Design review of the part built by this model. Coordinates are the model's own, in mm. Coordinates: 2 decimals unless noted, no trailing zeros. Loops run counter-clockwise (first coordinate to the right, second up) from the corner with the lowest first, then second, coordinate; pieces in that order, holes last. Notation, with made-up numbers: M 41.5,69 L 47.5,69 A12 cw 47.5,82 Z; hole C 13,50.5 d6. An arc over 180 degrees is marked long. Write item = value, one per line. Start each with the question number.
from build123d import *

# Parameters (mm, degrees)
SKETCH1_R               = 75.8825
BOSS_EXTRUDE1_DEPTH     = 38.1
SKETCH2_R               = 73.66
CUT_EXTRUDE1_DEPTH      = 101.6
SKETCH4_R               = 1.27
CUT_EXTRUDE3_DEPTH      = 76.8825
CUT_EXTRUDE3_DEPTH_BACK = 76.8825
SKETCH5_R               = 1.27
CUT_EXTRUDE4_DEPTH      = 76.8825001
CUT_EXTRUDE4_DEPTH_BACK = 76.8825001


with BuildPart() as part:
    # Sketch1 → Boss-Extrude1 (new body)
    with BuildSketch(Plane(origin=(0, 0, 0), x_dir=(1, 0, 0), z_dir=(0, 1, 0))):
        Circle(SKETCH1_R)
    extrude(amount=BOSS_EXTRUDE1_DEPTH)

    # Sketch2 → Cut-Extrude1 (cut)
    with BuildSketch(Plane(origin=(0, 38.1, 0), x_dir=(1, 0, 0), z_dir=(0, 1, 0))):
        Circle(SKETCH2_R)
    extrude(amount=-CUT_EXTRUDE1_DEPTH, mode=Mode.SUBTRACT)

    # Sketch4 → Cut-Extrude3 (cut, two sides)
    with BuildSketch(Plane(origin=(0, 0, 0), x_dir=(0, 0, -1), z_dir=(1, 0, 0))) as cut_extrude3_sk:
        with Locations((4.12e-07, 22.606)):
            Circle(SKETCH4_R)
        with Locations((4.12e-07, 15.494)):
            Circle(SKETCH4_R)
    extrude(amount=CUT_EXTRUDE3_DEPTH, mode=Mode.SUBTRACT)
    extrude(cut_extrude3_sk.sketch, amount=-CUT_EXTRUDE3_DEPTH_BACK, mode=Mode.SUBTRACT)

    # Sketch5 → Cut-Extrude4 (cut, two sides)
    with BuildSketch(Plane.XY) as cut_extrude4_sk:
        with Locations((7.8e-08, 15.493965738)):
            Circle(SKETCH5_R)
        with Locations((6.87e-07, 22.605965738)):
            Circle(SKETCH5_R)
    extrude(amount=CUT_EXTRUDE4_DEPTH, mode=Mode.SUBTRACT)
    extrude(cut_extrude4_sk.sketch, amount=-CUT_EXTRUDE4_DEPTH_BACK, mode=Mode.SUBTRACT)


solid = part.part
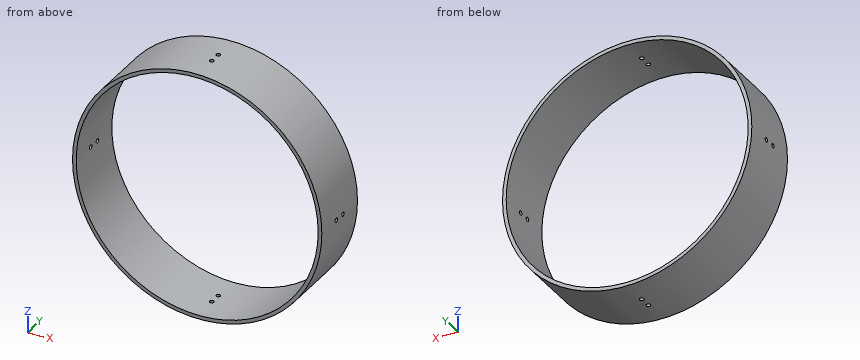
Q1. Add section B-B on x = -49.5. State the section outline as (y, z) points, plus the area to 3 significant figures.
Q2. Add section A-A on z = 6. State the section outline as (x, y) points.
Q3. Clearance check with flat-ended pins moving along their axes: P1, Ø8, axis at x = -54, y = 6.5, coming from the -Z side; P2, Ø10, axis at x = 53, y = 21, coming from the -Z side; P3, Ø5, axis at y = 18, z = 56, coming from the -X side. State where each tip first meets the part, or that it passes through.
Q4. To check wall thickness, follow line 1 (Y direction, x = -74, z = 0); line 2 (Z direction, x = 0, y = 8); line 3 (Z direction, x = -37, y = 32). State the ranges of each line that lie inside material, in increasing order. Write a range as from..to.
Q5. Add section C-C on y = 31.5. State the section outline as (x, z) points (1 decimal).
Values follow:
q1.outline = M 0,-57.51 L 38.1,-57.51 L 38.1,-54.55 L 0,-54.55 Z; M 0,54.55 L 38.1,54.55 L 38.1,57.51 L 0,57.51 Z
q1.area = 226 mm2
q2.outline = M -75.64,0 L -73.42,0 L -73.42,38.1 L -75.64,38.1 Z; M 73.42,0 L 75.64,0 L 75.64,38.1 L 73.42,38.1 Z
q3.P1 = -57.08
q3.P2 = -58.77
q3.P3 = -53.81
q4.line_1 = 0..14.22, 16.76..21.34, 23.88..38.1
q4.line_2 = -75.88..-73.66, 73.66..75.88
q4.line_3 = -66.25..-63.69, 63.69..66.25
q5.outline = C 0,0 d151.8; hole C 0,0 d147.3
